from build123d import *

# Parameters (mm, degrees)
BOSS_EXTRUDE1_DEPTH = 4.2
SKETCH2_R           = 1.550030902
CUT_EXTRUDE1_DEPTH  = 4.2
WASHER_DEPTH        = 0.5
SKETCH4_W           = 15.014396114
SKETCH4_H           = 18.830226703
CUT_EXTRUDE2_DEPTH  = 2.8


with BuildPart() as part:
    # Sketch1 → Boss-Extrude1 (new body)
    with BuildSketch(Plane(origin=(0, 0, 0), x_dir=(1, 0, 0), z_dir=(0, 1, 0))):
        with BuildLine():
            Line((-2.361421162, 16), (-3.343540366, 0.207937064))
            ThreePointArc((-3.343540366, 0.207937064), (0, -3.35), (3.343540366, 0.207937064))
            Line((3.343540366, 0.207937064), (2.361421162, 16))
            ThreePointArc((2.361421162, 16), (0, 18.361421162), (-2.361421162, 16))
        make_face()
    extrude(amount=BOSS_EXTRUDE1_DEPTH)

    # Sketch2 → Cut-Extrude1 (cut)
    with BuildSketch(Plane(origin=(0, 4.2, 0), x_dir=(1, 0, 0), z_dir=(0, 1, 0))):
        with Locations(Location((0, 0, 0), (0, 0, 270))):
            Circle(SKETCH2_R)
    extrude(amount=-CUT_EXTRUDE1_DEPTH, mode=Mode.SUBTRACT)

    # Sketch3 → Washer (add)
    with BuildSketch(Plane(origin=(0, 4.2, 0), x_dir=(1, 0, 0), z_dir=(0, 1, 0))):
        with BuildLine():
            Line((5.978845304, 9.183192045), (5.040969257, 11.241624252))
            ThreePointArc((5.040969257, 11.241624252), (2.163457141, 13.826055508), (5.039545151, 16.412071489))
            Line((5.039545151, 16.412071489), (5.976287141, 18.471020026))
            ThreePointArc((5.976287141, 18.471020026), (-0.036542776, 13.825449558), (5.978845304, 9.183192045))
        make_face()
    extrude(amount=WASHER_DEPTH)

    # Sketch4 → Cut-Extrude2 (cut)
    with BuildSketch(Plane(origin=(0, 0, 0), x_dir=(-1, 0, 0), z_dir=(0, -1, 0))):
        with Locations((-0.264298209, 12.569563008)):
            Rectangle(SKETCH4_W, SKETCH4_H)
    extrude(amount=-CUT_EXTRUDE2_DEPTH, mode=Mode.SUBTRACT)


solid = part.part
Read the model definition and answer for the solid it produces. Units are mm, in the model's axes. A direction names the side the tool comes from. Coordinates: 2 decimals unless noted, no trailing zeros. Order: outer loops, then holes, each group sorted by start corner. A loop starts at its lowest first (then second) coordinate and runs counter-clockwise, first axis right, second up. Notation, with made-up numbers: M 50,8.25 L 82,8.25 A26 cw 82,26.25 Z; hole C -19,40 d5. An arc over 180 degrees is marked long. Put each result on its own line as item: value. Start each with the question number.
Item 1: For faces 1 (the face through (2.97, 3, -6.24)), 2 (the face through (0, 1, -3.154)), 3 (the face through (5.516, 4.446, -10.198)), determine the directions among +Z, -Z, +X, -X, +Y, -Y from which every point of the face is accessible in a straight line to the end or side of a thin tool.
Item 2: Section B-B, the plane y = 0.6 is taken. Determine the outline of the cut face in (x, z).
Item 3: Given pin 1 Ø2 at (x, y) = (0.5, 0.5) entering from -Z; pin 2 Ø1.5 at (x, z) = (2, -12) entering from -Y; pin 3 Ø1.7 at (x, z) = (4, -11) entering from -Y, each flat-ended and moving along its own axis, determine where each tip first touches the part or whether it passes through.
Item 4: Consider probe 1 along Y at (x, z) = (-1.25, -4.75); probe 2 along Z at (x, y) = (0.5, 2.15); probe 3 along X at (y, z) = (1.5, 1). Determine where each line is inside the solid, lowest interval first. Write a range as [from, to].
Item 5: Section A-A, the plane z = 0 is taken. Determine the outline of the cut face in (x, y).
Item 6: Section D-D, the plane z = -14.5 is taken. Determine the outline of the cut face in (x, y), plus the area to 3 significant figures.
Item 7: Section C-C, the plane x = 5.25 is taken. Determine the outline of the cut face in (y, z), plus the area to 3 significant figures.
Computed:
1. face 1: -Z, +X, -Y
1. face 2: -Z, +X, -X, -Y
1. face 3: +X, +Y, -Y
2. outline: M -3.34,-0.21 L -3.16,-3.15 L 3.16,-3.15 L 3.34,-0.21 A3.35 ccw long Z; hole C 0,0 d3.1
3. pin 1: stops at z = -3.15
3. pin 2: stops at y = 2.8
3. pin 3: stops at y = 4.2
4. probe 1: y = [2.8, 4.2]
4. probe 2: z = [-3.15, -1.47], [1.47, 3.31]
4. probe 3: x = [-3.2, -1.18], [1.18, 3.2]
5. outline: M -3.35,0 L -1.55,0 L -1.55,4.2 L -3.35,4.2 Z; M 1.55,0 L 3.35,0 L 3.35,4.2 L 1.55,4.2 Z
6. outline: M -2.45,2.8 L 2.45,2.8 L 2.45,4.2 L 2.25,4.2 L 2.25,4.7 L 0.01,4.7 L 0.01,4.2 L -2.45,4.2 Z
6. area: 7.99 mm2
7. outline: M 4.2,-18.6 L 4.7,-18.6 L 4.7,-16.87 L 4.2,-16.87 Z; M 4.2,-10.78 L 4.7,-10.78 L 4.7,-9.05 L 4.2,-9.05 Z
7. area: 1.73 mm2
